Autodesk Inventor part; units mm, degrees
ref_plane "Work Plane1" through (0, 0, -15.5) normal (0, 0, 1) x (1, 0, 0)
ref_plane "YZ Plane" through (0, 0, 0) normal (1, 0, 0) x (0, 1, 0)
ref_plane "XZ Plane" through (0, 0, 0) normal (0, 1, 0) x (-1, 0, 0)
ref_plane "Work Plane1" through (0, 0, -15.5) normal (0, 0, 1) x (1, 0, 0)
sketch "Sketch1" plane through (0, 0, -15.5) normal (0, 0, 1) x (1, 0, 0)
  arc A0 (3.2082, 10) -> (16.2082, 10) centre (9.7082, 10) ccw
  line L0 (16.2082, 24) -> (16.2082, 10)
  line L1 (3.2082, 10) -> (3.2082, 24)
  arc A1 (16.2082, 24) -> (3.2082, 24) centre (9.7082, 24) ccw
extrude "Extrusion3" add sketch "Sketch1" along normal blind 1.5
sketch "Sketch2" plane through (0, 0, -14) normal (0, 0, 1) x (1, 0, 0)
  circle A0 centre (9.7082, 10) radius 2.5
extrude "Extrusion2" add sketch "Sketch2" along normal blind 1
sketch "Sketch3" plane through (0, 0, -14) normal (0, 0, 1) x (1, 0, 0)
  circle A0 centre (9.7082, 24) radius 2.5
extrude "Extrusion1" add sketch "Sketch3" along normal blind 1
hole "Hole2" at (9.7082, 10, -15.5) direction (0, 0, 1) diameter 3 depth 2.5
sketch "Sketch4" plane through (0, 0, -15.5) normal (0, 0, 1) x (1, 0, 0)
  point P0 (9.7082, 10)
hole "Hole1" at (9.7082, 24, -15.5) direction (0, 0, 1) diameter 3 depth 2.5
chamfer "Chamfer1" distance 1.5 angle 45 2 edges at (9.7082, 22.5, -15.5) (9.7082, 8.5, -15.5)
chamfer "Chamfer2" distance 1 angle 45 2 edges at (7.2082, 24, -14) (7.2082, 10, -14)
sketch "Sketch5" plane through (0, 0, -15.5) normal (0, 0, 1) x (1, 0, 0)
  point P0 (9.7082, 24)
properties part number "Belt Retainer"
Part model, mm, in its own coordinate system. A direction names the side the tool comes from. Round coordinates to 2 decimals unless told otherwise and drop trailing zeros. Order: outer loops, then holes, each group sorted by start corner. A loop starts at its lowest first (then second) coordinate and runs counter-clockwise, first axis right, second up. Notation, with made-up numbers: M 59.5,-30 L 79.5,-30 A11 ccw 79.5,-18 Z; hole C -4,9.25 d5. An arc over 180 degrees is marked long. Put each result on its own line as item: value. Start each with the question number.
1. Slice it at D-D on x = 5. List the corners of the cut face in (y, z), then the cut area to 3 significant figures.
2. Drill centre lines: probe 1 along Y at (x, z) = (9.5, -14.5); probe 2 along Y at (x, z) = (11.5, -14.9); probe 3 along X at (y, z) = (10, -13.5). Where is each one in solid material? Low to high. Write a range as [from, to].
3. Slice it at C-C on y = 16.25. List the corners of the cut face in (x, z).
4. Slice it at A-A on z = -14.75. List the corners of the cut face in (x, y).
5. Drop flat-ended pins along their axis: pin 1 (4 mm diameter, centred on x = 7, y = 13, fed in from +Z); pin 2 (1 mm diameter, centred on x = 6.5, y = 21, fed in from +Z); pin 3 (2.5 mm diameter, centred on x = 9.71, y = 24, fed in from +Z). Give the stop position or say it passes through.
6. Slice it at B-B on z = -13.45. List the corners of the cut face in (x, y).
7. Tool access for faces 1 (the face through (10, 17, -14)), 2 (the face through (10, 8, -13)): list every direction of +Z, -Z, +X, -X, +Y, -Y with a clear straight run to the whole face (end or side of a thin tool).
8. Two-plate mould, pull along Y, no slides. Class faces 3 (the face through (3.208, 17, -15)), 4 (the face through (9.85, 3.5, -14.76)), 5 (the face through (10.62, 8.81, -13.49)): +Y half, -Y half, draft (parallel to the pull), parting line (faces both ways), or undercut.
Findings:
1. outline: M 5.52,-15.5 L 28.48,-15.5 L 28.48,-14 L 5.52,-14 Z
1. area: 34.4 mm2
2. probe 1: [3.5, 8.01], [11.99, 22.01], [25.99, 30.5]
2. probe 2: [3.75, 8.4], [11.6, 22.4], [25.6, 30.25]
2. probe 3: [6.71, 8.21], [11.21, 12.71]
3. outline: M 3.21,-15.5 L 16.21,-15.5 L 16.21,-14 L 3.21,-14 Z
4. outline: M 3.21,10 A6.5 ccw 16.21,10 L 16.21,24 A6.5 ccw 3.21,24 Z; hole C 9.71,10 d4.5; hole C 9.71,24 d4.5
5. pin 1: z = -13
5. pin 2: z = -14
5. pin 3: through
6. outline: C 9.71,10 d5.9; C 9.71,24 d5.9; hole C 9.71,10 d3; hole C 9.71,24 d3
7. face 1: +Z
7. face 2: +Z, +X, -X, +Y, -Y
8. face 3: draft
8. face 4: -Y half
8. face 5: undercut
